Design review of the part built by this model. Coordinates are the model's own, in mm. Coordinates: 2 decimals unless noted, no trailing zeros. Write each loop counter-clockwise with the first axis right and the second up, starting at its lowest first coordinate (ties: lowest second). Pieces come first, ordered by that corner, then holes. Notation, with made-up numbers: (46, 22) - (86, 22) arc R13 cw to (86, 32) - close; hole circle Ø1 at (-1, 37.25). An arc over 180 degrees is marked (long way). Answer as CSV lines item,"result". Start each with the question number.
Q1. We need section C-C (z = 8.5). Write out the cut boundary in (x, y).
Q2. For line 1 along X through (y, z) = (2.5, 7); line 2 along Y through (x, z) = (0, 2.75); line 3 along Y through (x, z) = (243.2, 5.5), list the stretches that pass through material, from the lowest coordinate up. Write a range as [from, to].
Q3. We need section B-B (y = 0). Write out the cut boundary in (x, z).
Q4. Clearance check with flat-ended pins moving along their axes: pin 1 (1 mm diameter, centred on x = 135, z = 1.5, fed in from +Y); pin 2 (8 mm diameter, centred on x = 243.2, y = 0, fed in from -Z); pin 3 (1.5 mm diameter, centred on y = -6, z = 5.5, fed in from -X); pin 4 (4 mm diameter, centred on y = 6.5, z = 6, fed in from +X). State where each tip first meets the part, or that it passes through.
Q5. We need section A-A (x = 0). Write out the cut boundary in (y, z).
Q6. We need section D-D (x = 243.2). Write out the cut boundary in (y, z), plus the area to 3 significant figures.
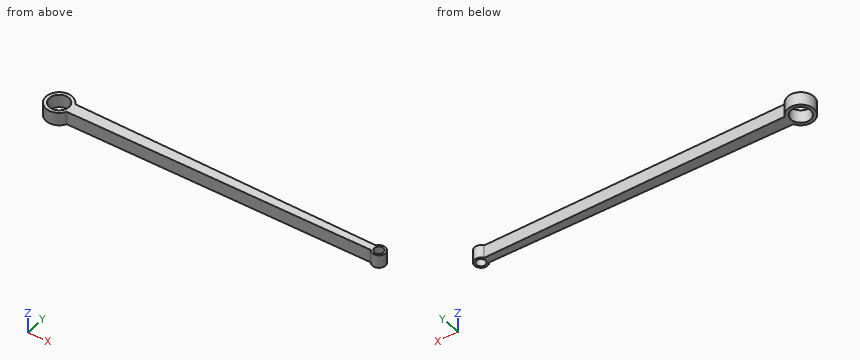
from build123d import *

# Parameters (mm, degrees)
ESBO_O1_R                = 7.5
ESBO_O1_R_2              = 3.5
RESSALTO_EXTRUS_O1_DEPTH = 10


with BuildPart() as part:
    # Esboço1 → Ressalto-extrusão1 (new body)
    with BuildSketch(Plane.XY):
        with BuildLine():
            Line((9.514211155, -4.507297718), (238.473101757, -2.705535542))
            ThreePointArc((238.473101757, -2.705535542), (238.91470232, -2.804462383), (239.267475736, -3.087920483))
            ThreePointArc((239.267475736, -3.087920483), (248.2, 0), (239.267475736, 3.087920483))
            ThreePointArc((239.267475736, 3.087920483), (238.91470232, 2.804462383), (238.473101757, 2.705535542))
            Line((238.473101757, 2.705535542), (9.514211155, 4.507297718))
            ThreePointArc((9.514211155, 4.507297718), (9.019006357, 4.643023372), (8.656436619, 5.006606142))
            ThreePointArc((8.656436619, 5.006606142), (-10, 0), (8.656436619, -5.006606142))
            ThreePointArc((8.656436619, -5.006606142), (9.019006357, -4.643023372), (9.514211155, -4.507297718))
        make_face()
        Circle(ESBO_O1_R, mode=Mode.SUBTRACT)
        with Locations((243.2, 0)):
            Circle(ESBO_O1_R_2, mode=Mode.SUBTRACT)
    extrude(amount=RESSALTO_EXTRUS_O1_DEPTH)


solid = part.part
Results list:
1,outline,"(8.66, -5.01) arc R1 cw to (9.51, -4.51) - (238.47, -2.71) arc R1 cw to (239.27, -3.09) arc R5 ccw (long way) to (239.27, 3.09) arc R1 cw to (238.47, 2.71) - (9.51, 4.51) arc R1 cw to (8.66, 5.01) arc R10 ccw (long way) to start; hole circle Ø15 at (0, 0); hole circle Ø7 at (243.2, 0)"
2,line 1,"x = [-9.68, -7.07], [7.07, 240.75], [245.65, 247.53]"
2,line 2,"y = [-10, -7.5], [7.5, 10]"
2,line 3,"y = [-5, -3.5], [3.5, 5]"
3,outline,"(-10, 0) - (-7.5, 0) - (-7.5, 10) - (-10, 10) - close; (7.5, 0) - (239.7, 0) - (239.7, 10) - (7.5, 10) - close; (246.7, 0) - (248.2, 0) - (248.2, 10) - (246.7, 10) - close"
4,pin 1,"stops at y = 3.52"
4,pin 2,"stops at z = 0"
4,pin 3,"stops at x = -8.51"
4,pin 4,"stops at x = 245.38"
5,outline,"(-10, 0) - (-7.5, 0) - (-7.5, 10) - (-10, 10) - close; (7.5, 0) - (10, 0) - (10, 10) - (7.5, 10) - close"
6,outline,"(-5, 0) - (-3.5, 0) - (-3.5, 10) - (-5, 10) - close; (3.5, 0) - (5, 0) - (5, 10) - (3.5, 10) - close"
6,area,"30.0 mm2"
